from build123d import *

# Parameters (mm, degrees)
SKETCH1_R           = 2
BOSS_EXTRUDE2_DEPTH = 2


with BuildPart() as part:
    # Sketch1 → Boss-Extrude2 (new body)
    with BuildSketch(Plane(origin=(0, 0, 0), x_dir=(1, 0, 0), z_dir=(0, 1, 0))):
        with BuildLine():
            Line((-33.676027055, 11.180582142), (15.211406628, 19.984204272))
            ThreePointArc((15.211406628, 19.984204272), (34.737966777, -7.78097648), (1.211790987, -13.090152535))
            ThreePointArc((1.211790987, -13.090152535), (-10.79582326, -5.653169844), (-24.912367612, -5.189826572))
            ThreePointArc((-24.912367612, -5.189826572), (-42.960314969, -4.320578887), (-33.676027055, 11.180582142))
        make_face()
        with Locations(Location((-33.676027055, 0.649629179, 0), (0, 0, 270))):
            Circle(SKETCH1_R, mode=Mode.SUBTRACT)
        with Locations(Location((-33.886225149, -5.846971221, 0), (0, 0, 270))):
            Circle(SKETCH1_R, mode=Mode.SUBTRACT)
        with Locations(Location((16.319944597, 0.014949315, 0), (0, 0, 270))):
            Circle(SKETCH1_R, mode=Mode.SUBTRACT)
        with Locations(Location((16.319944597, 15.014949315, 0), (0, 0, 270))):
            Circle(SKETCH1_R, mode=Mode.SUBTRACT)
        with BuildLine():
            Line((-32.205991929, 6.364880551), (-0.796707678, 12.021047159))
            ThreePointArc((-0.796707678, 12.021047159), (0.683130465, 8.373787285), (4.344424088, 6.929019304))
            Line((4.344424088, 6.929019304), (12.69431881, 2.108205339))
            ThreePointArc((12.69431881, 2.108205339), (12.133432549, 0.014949315), (12.69431881, -2.07830671))
            Line((12.69431881, -2.07830671), (6.575597959, -5.61095184))
            Line((6.575597959, -5.61095184), (2.986337283, -7.83499068))
            ThreePointArc((2.986337283, -7.83499068), (-11.570908116, -0.280369046), (-27.962567795, -0.827355859))
            ThreePointArc((-27.962567795, -0.827355859), (-28.59343775, 3.648360156), (-32.205991929, 6.364880551))
        make_face(mode=Mode.SUBTRACT)
        with BuildLine():
            Line((16.319944597, 4.201461363), (16.319944597, 11.266751624))
            ThreePointArc((16.319944597, 11.266751624), (21.945845752, 9.759295953), (26.064291236, 5.64085047))
            Line((26.064291236, 5.64085047), (19.945570385, 2.108205339))
            ThreePointArc((19.945570385, 2.108205339), (18.413200622, 3.640575102), (16.319944597, 4.201461363))
        make_face(mode=Mode.SUBTRACT)
        with BuildLine():
            Line((19.945570385, -2.07830671), (26.064291236, -5.61095184))
            ThreePointArc((26.064291236, -5.61095184), (21.945845752, -9.729397324), (16.319944597, -11.236852995))
            Line((16.319944597, -11.236852995), (16.319944597, -4.171562734))
            ThreePointArc((16.319944597, -4.171562734), (18.413200622, -3.610676472), (19.945570385, -2.07830671))
        make_face(mode=Mode.SUBTRACT)
        with BuildLine():
            ThreePointArc((2.244741471, 12.762469116), (2.384407332, 9.940848466), (5.206027982, 10.080514326))
            ThreePointArc((5.206027982, 10.080514326), (5.413174271, 10.304609299), (5.624838222, 10.524442221))
            ThreePointArc((5.624838222, 10.524442221), (6.978596806, 11.744142082), (8.470307193, 12.790626759))
            ThreePointArc((8.470307193, 12.790626759), (8.519771502, 12.820887047), (8.569352462, 12.850955823))
            ThreePointArc((8.569352462, 12.850955823), (9.246853, 15.59359008), (6.504218744, 16.271090618))
            ThreePointArc((6.504218744, 16.271090618), (6.441427011, 16.233010062), (6.378783011, 16.194686965))
            ThreePointArc((6.378783011, 16.194686965), (4.489608616, 14.869368007), (2.775143075, 13.324680936))
            ThreePointArc((2.775143075, 13.324680936), (2.50708158, 13.046273859), (2.244741471, 12.762469116))
        make_face(mode=Mode.SUBTRACT)
    extrude(amount=BOSS_EXTRUDE2_DEPTH)


solid = part.part
Model file for the job. Use its own axes, mm. A direction names the side the tool comes from. Give positions to 0.01 mm unless a question says otherwise; leave off trailing zeros. Order: outer loops, then holes, each group sorted by start corner. A loop starts at its lowest first (then second) coordinate and runs counter-clockwise, first axis right, second up. Notation, with made-up numbers: (-32, 79) - (19, 79) arc R22 cw to (19, 118) - close; hole circle Ø4 at (38.25, 69). An arc over 180 degrees is marked (long way). One line per item, written item: value.
Item 1: Slice it at B-B (x = 7.5). List the corners of the cut face in (y, z), then the cut area to 3 significant figures.
Response values:
outline: (0, -18.6) - (2, -18.6) - (2, -16.56) - (0, -16.56) - close; (0, -12.14) - (2, -12.14) - (2, -5.11) - (0, -5.11) - close; (0, 5.08) - (2, 5.08) - (2, 17.94) - (0, 17.94) - close
area: 43.9 mm2
Item 2: Slice it at C-C (y = 0.75). Give the number of separate pieces and of enclosed holes in the cut face, then the cut area to 3 significant figures.
Response values:
separate pieces: 1
enclosed holes: 8
area: 1,470 mm2
Item 3: Slice it at A-A (x = -13.5). List the corners of the cut face in (y, z), then the cut area to 3 significant figures.
Response values:
outline: (0, -14.81) - (2, -14.81) - (2, -9.73) - (0, -9.73) - close; (0, -0.1) - (2, -0.1) - (2, 4.98) - (0, 4.98) - close
area: 20.3 mm2
Item 4: Two-plate mould, pull along Z, no slides. Class faces 1 (the cylindrical face through (-42.81, 0.99, 4.59)), 2 (the flat face through (22.96, 0.99, 3.82)), 3 (the cylindrical face through (-10.605, 0.986, 5.712)): released by +Z, released by -Z, zero draft, split by the parting line, or undercut.
Response values:
face 1: split by the parting line
face 2: undercut
face 3: released by +Z
Item 5: Pin check, flat tips, straight feed: pin 1 Ø0.6 at (y, z) = (1.5, 7.5) entering from +X; pin 2 Ø3 at (x, z) = (21.5, 12) entering from -Y. Stop position of each tip, or through.
Response values:
pin 1: x = 34.97
pin 2: y = 0
Item 6: Tool access for faces 4 (the flat face through (-3, 2, 4)), 5 (the cylindrical face through (12.134, 0.986, -0.046)): list every direction of +Z, -Z, +X, -X, +Y, -Y with a clear straight run to the whole face (end or side of a thin tool).
Response values:
face 4: +Z, -Z, +X, -X, +Y
face 5: +Y, -Y
Item 7: Wall check: line 1 (Z direction, x = 9, y = 1); line 2 (X direction, y = 0.6, z = -5); line 3 (X direction, y = 0.8, z = 6.5). Give the ranges that are in metal, low to high.
Response values:
line 1: -18.87 to -15.92, -13.2 to -4.24, 4.21 to 18.6
line 2: -43.27 to -29.69, 7.69 to 16.32, 24.95 to 35.69
line 3: -41.41 to -35.78, -32 to -25.94, -8.4 to 1.41, 5.14 to 16.32, 25.49 to 35.23
